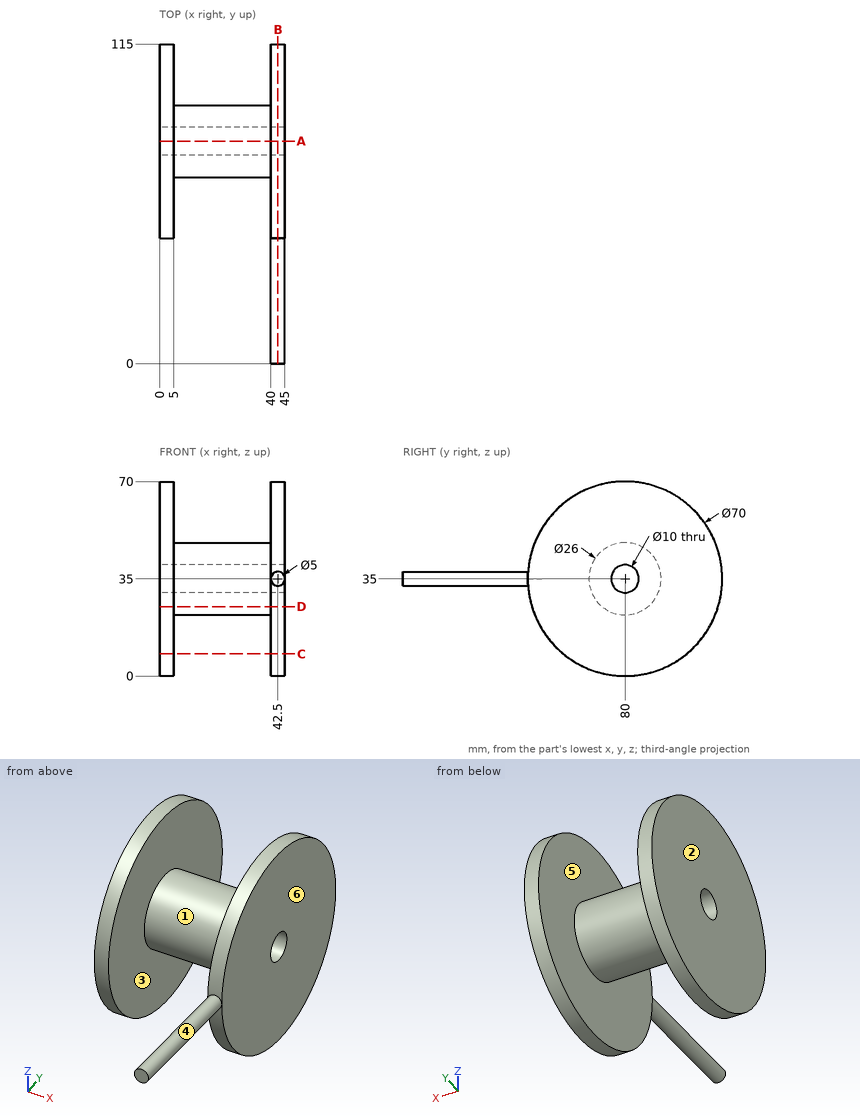
Input: dimensioned drawing with shaded views. Units: mm. Origin: part minimum x, y, z. A direction names the side the tool comes from. Give positions to 0.01 mm unless a question says otherwise; leave off trailing zeros. Loops run counter-clockwise (first coordinate to the right, second up) from the corner with the lowest first, then second, coordinate; pieces in that order, holes last. Notation, with made-up numbers: M 79.25,-18 L 110.25,-18 A21 ccw 110.25,18 Z; hole C 41,13 d9. An arc over 180 degrees is marked long. Put each result on its own line as item: value. Start each with the question number.
1) Pull-direction query (X, two-part tool) for the marked faces 3, 4, 5 and 6; classes: pulls with the +X half, pulls with the -X half, needs draft (parallel to the pull), parting line crosses it, or undercut.
2) Cut plane C-C (z = 8). Output: boundary loops of the cut face in (x, y), then the cut area to 3 significant figures.
3) Access query for the marked faces 1 and 2. Directions: +Z, -Z, +X, -X, +Y, -Y. A direction counts if a zero-diameter tool reaches every point of the face in a straight line with its end or side. Return the directions, or none.
4) Cut plane A-A (y = 80). Output: boundary loops of the cut face in (x, z), then the cut area to 3 significant figures.
5) Cut plane B-B (x = 42.5). Output: boundary loops of the cut face in (y, z).
6) Cut plane D-D (z = 25). Output: boundary loops of the cut face in (x, y), then the cut area to 3 significant figures.
7) Ray query, line 1 along Y through (x, z) = (34, 35); line 2 along X through (y, z) = (93, 63.5); line 3 along Y through (x, z) = (18, 23). Return the intervals inside material, ascending.
8) Contact query for a flat-ended pin moving along its axis: pin 1 (5 mm diameter, centred on x = 40.5, y = 45.5, fed in from +Z). Output: stop coordinate, or through.
Verdict:
1. face 3: undercut
1. face 4: parting line crosses it
1. face 5: undercut
1. face 6: pulls with the +X half
2. outline: M 0,57.73 L 5,57.73 L 5,102.27 L 0,102.27 Z; M 40,57.73 L 45,57.73 L 45,102.27 L 40,102.27 Z
2. area: 445 mm2
3. face 1: none
3. face 2: +Z, -Z, -X, +Y, -Y
4. outline: M 0,0 L 5,0 L 5,22 L 40,22 L 40,0 L 45,0 L 45,30 L 0,30 Z; M 0,40 L 45,40 L 45,70 L 40,70 L 40,48 L 5,48 L 5,70 L 0,70 Z
4. area: 1,160 mm2
5. outline: M 0,32.5 L 45.09,32.5 A35 ccw long 45.09,37.5 L 0,37.5 Z; hole C 80,35 d10
6. outline: M 0,46.46 L 5,46.46 L 5,71.69 L 40,71.69 L 40,46.46 L 45,46.46 L 45,113.54 L 40,113.54 L 40,88.31 L 5,88.31 L 5,113.54 L 0,113.54 Z
6. area: 1,250 mm2
7. line 1: 67 to 75, 85 to 93
7. line 2: 0 to 5, 40 to 45
7. line 3: 75 to 85
8. pin 1: z = 49.18
